Part model, mm, in its own coordinate system. A direction names the side the tool comes from. Coordinates: 2 decimals unless noted, no trailing zeros. Write each loop counter-clockwise with the first axis right and the second up, starting at its lowest first coordinate (ties: lowest second). Pieces come first, ordered by that corner, then holes. Notation, with made-up numbers: (65.5, 40) - (97.5, 40) arc R25 ccw to (97.5, 75) - close; hole circle Ø10 at (52, 18). An arc over 180 degrees is marked (long way). Write each question's results on one line, items separated by ' | '.
from build123d import *

# Parameters (mm, degrees)
SKETCH_1_R               = 2.5
EXTRUDE_1_DEPTH          = 38.5
CUT_EXTRUDE_1_DEPTH      = 39.661996844
CUT_EXTRUDE_1_DEPTH_BACK = 39.661996844
CUT_EXTRUDE_2_DEPTH      = 39.661996957
CUT_EXTRUDE_2_DEPTH_BACK = 39.661996957
SKETCH_3_W               = 1.5
SKETCH_3_H               = 6


with BuildPart() as part:
    # 草图1 → 凸台-拉伸1 (new body)
    with BuildSketch(Plane(origin=(0, 0, 0), x_dir=(1, 0, 0), z_dir=(0, 1, 0))):
        with Locations(Location((0, 0, 0), (0, 0, 270))):
            Circle(SKETCH_1_R)
    extrude(amount=EXTRUDE_1_DEPTH)

    # 草图2 → 切除-拉伸1 (cut, two sides: drawn at the far end of the back side and taken through both)
    with BuildSketch(Plane.XY.offset(-CUT_EXTRUDE_1_DEPTH_BACK)):
        with BuildLine():
            ThreePointArc((-2.5, 36), (-1.767766953, 37.767766953), (0, 38.5))
            Line((0, 38.5), (-2.5, 38.5))
            Line((-2.5, 38.5), (-2.5, 36))
        make_face()
        with BuildLine():
            Line((2.5, 38.5), (0, 38.5))
            ThreePointArc((0, 38.5), (1.767766953, 37.767766953), (2.5, 36))
            Line((2.5, 36), (2.5, 38.5))
        make_face()
        with BuildLine():
            ThreePointArc((1.5, 36), (1.060660172, 37.060660172), (0, 37.5))
            Line((0, 37.5), (0, 34.5))
            ThreePointArc((0, 34.5), (1.060660172, 34.939339828), (1.5, 36))
        make_face()
        with BuildLine():
            Line((0, 34.5), (0, 37.5))
            ThreePointArc((0, 37.5), (-1.5, 36), (0, 34.5))
        make_face()
    extrude(amount=CUT_EXTRUDE_1_DEPTH + CUT_EXTRUDE_1_DEPTH_BACK, mode=Mode.SUBTRACT)

    # 草图3 → 切除-拉伸2 (cut, two sides: drawn at the far end of the back side and taken through both)
    with BuildSketch(Plane(origin=(0, 0, 0), x_dir=(0, 0, -1), z_dir=(1, 0, 0)).offset(-CUT_EXTRUDE_2_DEPTH_BACK)):
        with Locations((-1.75, 35.5)):
            Rectangle(SKETCH_3_W, SKETCH_3_H)
        with Locations((1.75, 35.5)):
            Rectangle(SKETCH_3_W, SKETCH_3_H)
    extrude(amount=CUT_EXTRUDE_2_DEPTH + CUT_EXTRUDE_2_DEPTH_BACK, mode=Mode.SUBTRACT)


solid = part.part
(1) Saw through at C-C on z = 1.95. Write the cut outline in (x, y).
Return value:
outline: (-1.56, 0) - (1.56, 0) - (1.56, 32.5) - (-1.56, 32.5) - close
(2) Wall check: line 1 (Y direction, x = 0.7, z = -2); line 2 (Z direction, x = -0.3, y = 34); line 3 (Y direction, x = -0.4, z = 0.25). Give the ranges that are in metal, low to high. Write a range as from..to.
Return value:
line 1: y = 0..32.5 | line 2: z = -1..1 | line 3: y = 0..34.55, 37.45..38.47
(3) Saw through at B-B on y = 23.5. Write the cut outline in (x, z).
Return value:
outline: circle Ø5 at (0, 0)
(4) 3-axis set-ups, long thin cutter, end or side, ignore diameter. For faces 1 (the flat face through (0, 32.5, -2)), 2 (the flat face through (0, 34, 1)), 3 (the flat face through (0, 0, 0)): which of +Z, -Z, +X, -X, +Y, -Y reach the whole face in a straight line?
Return value:
face 1: -Z, +X, -X, +Y | face 2: +Z, +X, -X, +Y | face 3: +Z, -Z, +X, -X, -Y
(5) Saw through at A-A on z = 0. Write the cut outline in (x, y).
Return value:
outline: (-2.5, 0) - (2.5, 0) - (2.5, 36) arc R2.5 ccw to (-2.5, 36) - close; hole circle Ø3 at (0, 36)
(6) Flat gauge pins, fed straight in: P1, Ø1.2, axis at x = -0.5, z = 2, coming from the +Y side; P2, Ø1, axis at x = -1, z = -0.5, coming from the +Y side. Where does each tip first touch, or does it go through?
Return value:
P1: stops at y = 32.5 | P2: stops at y = 38.45
